CAD build for the part. Positions are in the model's coordinates, mm. A direction names the side the tool comes from. Give positions to 0.01 mm unless a question says otherwise; leave off trailing zeros. Write each loop counter-clockwise with the first axis right and the second up, starting at its lowest first coordinate (ties: lowest second). Pieces come first, ordered by that corner, then holes. Notation, with made-up numbers: M -25,61.25 L 18,61.25 A10 ccw 18,76.25 Z; hole C -0.75,60 d8. An arc over 180 degrees is marked long. One line per question, with ' | ' between items. Start each with the question number.
1. Which spindle directions (+Z, -Z, +X, -X, +Y, -Y) get a long thin tool onto all of the face, cutting with end or side? Do faces 4 (the face through (112, 12, 4)), 5 (the face through (101, 5, 4)), 6 (the face through (5.58, 21.17, 4.26)). Say none if no direction does.
2. Pull direction Z, two halves, no side cores. Call faces 1 (the face through (106.58, 18.83, 4.26)), 2 (the face through (0, 12, 4)), 3 (the face through (55, 13, 0)): released by +Z, released by -Z, zero draft, split by the parting line, or undercut.
3. Wall check: L1, parallel to Y at x = 105, z = 4; L2, parallel to Y at x = 6.5, z = 5; L3, parallel to X at y = 20.5, z = 4.5. Give the ranges that are in metal, low to high.
4. Cut at B-B, the plane y = 20. Write the cut outline in (x, z), then the cut area to 3 significant figures.
5. Cut at A-A, the plane z = 4. Write the cut outline in (x, y), then the cut area to 3 significant figures.
6. Flat gauge pins, fed straight in: pin 1 (0.7 mm diameter, centred on y = 5, z = 4, fed in from +X); pin 2 (2 mm diameter, centred on y = 20, z = 4, fed in from -X). Where does each tip first touch, or does it go through?
```python
from build123d import *

# Parameters (mm, degrees)
ESQUISSE1_W             = 112
ESQUISSE1_H             = 25
BASE_EXTRUSION_DEPTH    = 8
ESQUISSE2_R             = 1.2
ENL_V_MAT_EXTRU_1_DEPTH = 11
ENL_V_START             = -11
ESQUISSE3_R             = 1.2
ENL_V_MAT_EXTRU_2_DEPTH = 11


with BuildPart() as part:
    # Esquisse1 → Base-Extrusion (new body)
    with BuildSketch(Plane.XY):
        with Locations((56, 12.5)):
            Rectangle(ESQUISSE1_W, ESQUISSE1_H)
    extrude(amount=BASE_EXTRUSION_DEPTH)

    # Esquisse2 → Enlèv. mat.-Extru.1 (cut)
    with BuildSketch(Plane(origin=(112, 0, 0), x_dir=(0, 0, -1), z_dir=(1, 0, 0))):
        with Locations((-4, 20)):
            Circle(ESQUISSE2_R)
        with Locations((-4, 5)):
            Circle(ESQUISSE2_R)
    extrude(amount=-ENL_V_MAT_EXTRU_1_DEPTH, mode=Mode.SUBTRACT)

    # Esquisse3 → Enlèv. mat.-Extru.2 (cut)
    with BuildSketch(Plane.ZY.offset(ENL_V_START)):
        with Locations(Location((4, 20, 0), (0, 0, 180))):
            Circle(ESQUISSE3_R)
        with Locations(Location((4, 5, 0), (0, 0, 180))):
            Circle(ESQUISSE3_R)
    extrude(amount=ENL_V_MAT_EXTRU_2_DEPTH, mode=Mode.SUBTRACT)


solid = part.part
```
Here are the results:
1) face 4: +Z, -Z, +X, +Y, -Y | face 5: +X | face 6: -X
2) face 1: undercut | face 2: zero draft | face 3: released by -Z
3) L1: 0 to 3.8, 6.2 to 18.8, 21.2 to 25 | L2: 0 to 4.34, 5.66 to 19.34, 20.66 to 25 | L3: 11 to 101
4) outline: M 0,0 L 112,0 L 112,2.8 L 101,2.8 L 101,5.2 L 112,5.2 L 112,8 L 0,8 L 0,5.2 L 11,5.2 L 11,2.8 L 0,2.8 Z | area: 843 mm^2
5) outline: M 0,0 L 112,0 L 112,3.8 L 101,3.8 L 101,6.2 L 112,6.2 L 112,18.8 L 101,18.8 L 101,21.2 L 112,21.2 L 112,25 L 0,25 L 0,21.2 L 11,21.2 L 11,18.8 L 0,18.8 L 0,6.2 L 11,6.2 L 11,3.8 L 0,3.8 Z | area: 2,690 mm^2
6) pin 1: x = 101 | pin 2: x = 11
